Study the drawing (mm; zero at the part's minimum x, y, z) and answer. A direction names the side the tool comes from. Coordinates: 2 decimals unless noted, no trailing zeros. Loops run counter-clockwise (first coordinate to the right, second up) from the corner with the lowest first, then second, coordinate; pieces in that order, holes last. Notation, with made-up numbers: (-26, 29) -> (-9, 29) arc R17 cw to (-9, 49) -> close; hole circle Ø5 at (4.5, 60). An arc over 180 degrees is marked (long way). One line per question, with ' | ' between items. Start each with the question number.
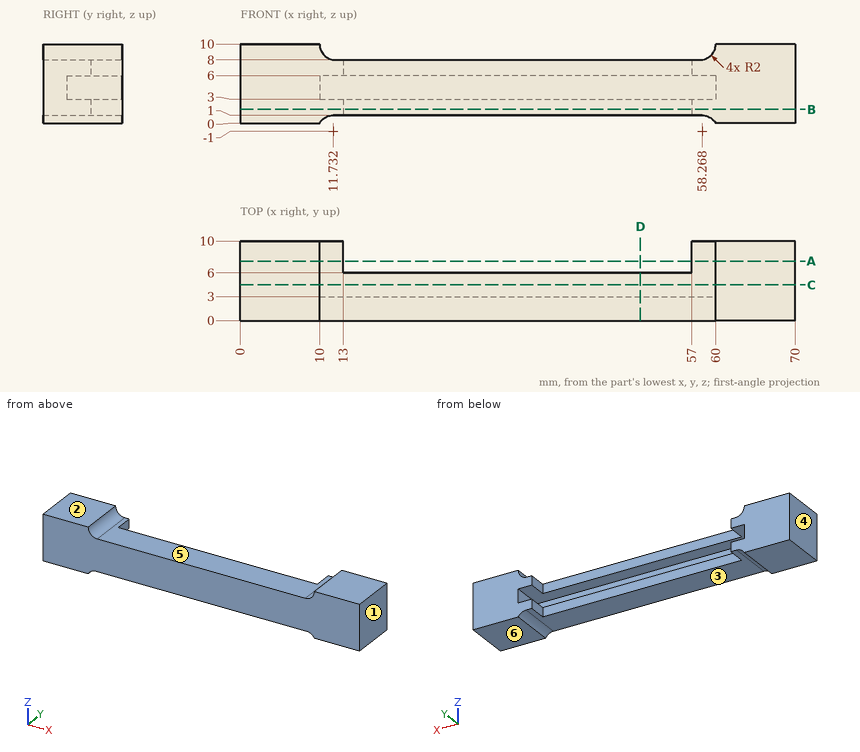
(1) Section B-B on z = 1.75 is taken. Write down the section's boundary in (x, y), plus the area to 3 significant figures.
(2) Find the intervals of material crossed by probe 1 along Z at (x, y) = (23, 4.5); probe 2 along X at (y, z) = (9.75, 5.75); probe 3 along Y at (x, z) = (50, 6.25), in increasing order. Write a range as from..to.
(3) Determine the mould class of the marked faces 1, 2, 3 and 4 for opening direction X: +X half, -X half, draft (parallel to the pull), parting line (faces both ways), or undercut.
(4) Section D-D on x = 50.5 is taken. Write down the section's boundary in (y, z).
(5) Each of these flat-tipped pins is pushed along its axis until it touches: pin 1 Ø2 at (x, y) = (46, 5) entering from -Z; pin 2 Ø2.5 at (x, z) = (31.5, 4) entering from +Y; pin 3 Ø2 at (x, y) = (31.5, 2) entering from +Z. Where does it stop, or does it pass through?
(6) Section A-A on y = 7.5 is taken. Write down the section's boundary in (x, z), plus the area to 3 significant figures.
(7) A tool of negligible diameter and unlimited length cuts with its end or side. For the marked faces 5 and 6, from which of +Z, -Z, +X, -X, +Y, -Y can it reach the whole face along a straight path? Write none if from no direction.
(8) Section C-C on y = 4.5 is taken. Write down the section's boundary in (x, z), plus the area to 3 significant figures.
Working result:
1) outline: (0, 0) -> (70, 0) -> (70, 10) -> (57, 10) -> (57, 6) -> (13, 6) -> (13, 10) -> (0, 10) -> close | area: 524 mm2
2) probe 1: z = 1..3, 6..8 | probe 2: x = 0..10, 60..70 | probe 3: y = 0..6
3) face 1: +X half | face 2: draft | face 3: undercut | face 4: -X half
4) outline: (0, 1) -> (6, 1) -> (6, 3) -> (3, 3) -> (3, 6) -> (6, 6) -> (6, 8) -> (0, 8) -> close
5) pin 1: stops at z = 1 | pin 2: stops at y = 6 | pin 3: stops at z = 8
6) outline: (0, 0) -> (10, 0) arc R2 cw to (11.73, 1) -> (13, 1) -> (13, 3) -> (10, 3) -> (10, 6) -> (13, 6) -> (13, 8) -> (12, 8) arc R2 cw to (10, 10) -> (0, 10) -> close; (57, 1) -> (58.27, 1) arc R2 cw to (60, 0) -> (70, 0) -> (70, 10) -> (60, 10) arc R2 cw to (58, 8) -> (57, 8) -> (57, 6) -> (60, 6) -> (60, 3) -> (57, 3) -> close | area: 227 mm2
7) face 5: +Z, +Y, -Y | face 6: -Z, +X, -X, +Y, -Y
8) outline: (0, 0) -> (10, 0) arc R2 cw to (11.73, 1) -> (58.27, 1) arc R2 cw to (60, 0) -> (70, 0) -> (70, 10) -> (60, 10) arc R2 cw to (58, 8) -> (12, 8) arc R2 cw to (10, 10) -> (0, 10) -> close; hole (10, 3) -> (60, 3) -> (60, 6) -> (10, 6) -> close | area: 403 mm2
